```python
from build123d import *

# Parameters (mm, degrees)
EXTRUDE_1_DEPTH     = 3
SKETCH_2_R          = 2.1
CUT_EXTRUDE_1_DEPTH = 39
CUT_EXTRUDE_2_DEPTH = 10
EXTRUDE_4_DEPTH     = 3
FILLET_1_R          = 4
FILLET_2_R          = 4


with BuildPart() as part:
    # Эскиз1 → Бобышка-Вытянуть1 (new body)
    with BuildSketch(Plane.XY):
        Polygon((0, 0), (0, 140), (230, -20), (230, -60), (200, -60), align=None)
    extrude(amount=EXTRUDE_1_DEPTH)

    # Эскиз2 → Вырез-Вытянуть1 (cut)
    with BuildSketch(Plane.XY.offset(3)):
        with Locations((10, 75)):
            Circle(SKETCH_2_R)
        with Locations((10, 120.2)):
            Circle(SKETCH_2_R)
    extrude(amount=-CUT_EXTRUDE_1_DEPTH, mode=Mode.SUBTRACT)

    # Эскиз5 → Вырез-Вытянуть2 (cut)
    with BuildSketch(Plane.XY.offset(3)):
        Polygon((220, -19.134315533), (220, -55), (200.733844182, -55), (20, -0.779846746), (20, 119.99611925), align=None)
    extrude(amount=-CUT_EXTRUDE_2_DEPTH, mode=Mode.SUBTRACT)

    # Эскиз7 → Бобышка-Вытянуть4 (add)
    with BuildSketch(Plane.XY):
        Polygon((105.308657106, -23.240351925), (126.380835381, -29.562005407), (142.759664858, 25.034092851), (121.687486583, 31.355746333), (106.745396534, -18.451220499), (99.082786252, -16.152437414), (107.752824145, 12.747688898), (20, 55.165339274), (20, 64.05093323), (110.080901053, 20.507945256), (118.313419369, 47.949672977), (20, 116.341616886), (20, 126.086956522), (220.176468292, -13.166238812), (220.176468292, -22.911578447), (151.136541271, 25.116196871), (134.043445663, -31.860788492), (201.17415069, -52), (220, -52), (220, -55), (200.733844182, -55), (20, -0.779846746), (20, 2.352245207), (97.646046824, -20.94156884), align=None)
    extrude(amount=EXTRUDE_4_DEPTH)

    # Скругление1
    fillet_1_edges = [part.edges().sort_by_distance(p)[0] for p in [
        (0, 0, 1.5),
        (0, 140, 1.5),
        (230, -20, 1.5),
        (230, -60, 1.5),
        (200, -60, 1.5),
    ]]
    fillet(fillet_1_edges, radius=FILLET_1_R)

    # Скругление2
    fillet_2_edges = [part.edges().sort_by_distance(p)[0] for p in [
        (220, -22.788817896, 1.5),
        (151.136541271, 25.116196871, 1.5),
        (20, 2.352245207, 1.5),
        (220, -52, 1.5),
        (201.17415069, -52, 1.5),
        (134.043445663, -31.860788492, 1.5),
        (20, 116.341616886, 1.5),
        (118.313419369, 47.949672977, 1.5),
        (110.080901053, 20.507945256, 1.5),
        (20, 64.05093323, 1.5),
        (20, 55.165339274, 1.5),
        (107.752824145, 12.747688898, 1.5),
        (121.687486583, 31.355746333, 1.5),
        (142.759664858, 25.034092851, 1.5),
        (126.380835381, -29.562005407, 1.5),
    ]]
    fillet(fillet_2_edges, radius=FILLET_2_R)


solid = part.part
```
Build history of the part. All positions in model axes, mm. A direction names the side the tool comes from. Coordinates: 2 decimals unless noted, no trailing zeros. Order: outer loops, then holes, each group sorted by start corner. A loop starts at its lowest first (then second) coordinate and runs counter-clockwise, first axis right, second up. Notation, with made-up numbers: M 55,6 L 98,6 A27 cw 98,44 Z; hole C 50.25,-32.5 d10. An arc over 180 degrees is marked long. One line per question, with ' | ' between items. Start each with the question number.
1. Cut at B-B (y = 56.5). Write the cut outline in (x, z).
2. Tool access for faces 1 (the face through (63.47, 43.04, 1.48)), 2 (the face through (90, 24, 3)): list every direction of +Z, -Z, +X, -X, +Y, -Y with a clear straight run to the whole face (end or side of a thin tool).
3. Mould opens along Y. For faces 3 (the face through (114.4, 34.9, 1.5)), 4 (the face through (102.52, -30.756, 1.479)), 5 (the face through (90, 24, 0)) say: +Y half, -Y half, draft (parallel to the pull), parting line (faces both ways), or undercut.
4. Cut at C-C (x = 213.5). Write the cut outline in (y, z), plus the area to 3 significant figures.
5. Cut at D-D (y = -3.5). Write the cut outline in (x, z), plus the area to 3 significant figures.
6. Wall check: line 1 along Y through (x, z) = (64, 2.05); line 2 along Y through (x, z) = (42, 2.5); line 3 along Y through (x, z) = (219, 0.2). Give the ranges that are in metal, low to high. Write a range as [from, to].
7. Cut at A-A (x = 56.5). Write the cut outline in (y, z), plus the area to 3 significant figures.
8. Flat gauge pins, fed straight in: P1, Ø3.5, axis at x = 10, y = 75, coming from the +Z side; P2, Ø1, axis at x = 35.5, z = 1.5, coming from the +Y side; P3, Ø6.5, axis at x = 10, y = 120.2, coming from the -Z side; P4, Ø1.5, axis at x = 208, z = 2, coming from the +Y side. Where does each tip first touch, or does it go through?
The answers:
1) outline: M 0,0 L 35.62,0 L 35.62,3 L 0,3 Z; M 106.02,0 L 120.03,0 L 120.03,3 L 106.02,3 Z
2) face 1: +Z, -Z | face 2: +Z, +X, -X, +Y, -Y
3) face 3: undercut | face 4: -Y half | face 5: draft
4) outline: M -60,0 L -52,0 L -52,3 L -60,3 Z; M -18.27,0 L -8.52,0 L -8.52,3 L -18.27,3 Z | area: 53.2 mm2
5) outline: M 11.67,0 L 39.51,0 L 39.51,3 L 11.67,3 Z; M 102.88,0 L 111.23,0 L 111.23,3 L 102.88,3 Z; M 134.2,0 L 142.55,0 L 142.55,3 L 134.2,3 Z; M 192.27,0 L 206.28,0 L 206.28,3 L 192.27,3 Z | area: 176 mm2
6) line 1: y = [-19.2, -10.85], [33.9, 42.78], [85.73, 95.48] | line 2: y = [-12.6, -4.25], [44.53, 53.42], [101.04, 110.78] | line 3: y = [-60, -50.65], [-22.23, -12.35]
7) outline: M -16.95,0 L -8.6,0 L -8.6,3 L -16.95,3 Z; M 37.52,0 L 46.41,0 L 46.41,3 L 37.52,3 Z; M 90.95,0 L 100.7,0 L 100.7,3 L 90.95,3 Z | area: 80.9 mm2
8) P1: passes through | P2: stops at y = 115.65 | P3: stops at z = 0 | P4: stops at y = -4.17
